```python
from build123d import *

# Parameters (mm, degrees)
SKETCH_1_R       = 1.25
BOARD_DEPTH      = 1
SKETCH_2_W       = 37.3
SKETCH_2_H       = 30
SCREEN_DEPTH     = 2
SCREEN_RADIUS_R  = 3.5
SKETCH_3_W       = 51
SKETCH_3_H       = 5
PLUG_DEPTH       = 7
SKETCH_4_W       = 15.14
SKETCH_4_H       = 20
SPEAKER_DEPTH    = 5
SKETCH_5_W       = 4.5
SKETCH_5_H       = 2.5
BUTTON_DEPTH     = 3.4
SKETCH_6_R       = 1
BUTTON_TAP_DEPTH = 0.5


with BuildPart() as part:
    # 草图1 → board (new body)
    with BuildSketch(Plane(origin=(0, 0, 0), x_dir=(1, 0, 0), z_dir=(0, 1, 0))):
        with BuildLine():
            Line((-29.5, 15), (29.5, 15))
            ThreePointArc((29.5, 15), (31.621320344, 14.121320344), (32.5, 12))
            Line((32.5, 12), (32.5, -12))
            ThreePointArc((32.5, -12), (31.621320344, -14.121320344), (29.5, -15))
            Line((29.5, -15), (-29.5, -15))
            ThreePointArc((-29.5, -15), (-31.621320344, -14.121320344), (-32.5, -12))
            Line((-32.5, -12), (-32.5, 12))
            ThreePointArc((-32.5, 12), (-31.621320344, 14.121320344), (-29.5, 15))
        make_face()
        with Locations(Location((-29.5, 12, 0), (0, 0, 270))):
            Circle(SKETCH_1_R, mode=Mode.SUBTRACT)
        with Locations(Location((29.5, 12, 0), (0, 0, 270))):
            Circle(SKETCH_1_R, mode=Mode.SUBTRACT)
        with Locations(Location((-29.5, -12, 0), (0, 0, 270))):
            Circle(SKETCH_1_R, mode=Mode.SUBTRACT)
        with Locations(Location((29.5, -12, 0), (0, 0, 270))):
            Circle(SKETCH_1_R, mode=Mode.SUBTRACT)
    extrude(amount=BOARD_DEPTH)

    # 草图2 → screen (add)
    with BuildSketch(Plane(origin=(0, 1, 0), x_dir=(1, 0, 0), z_dir=(0, 1, 0))):
        with Locations((-8.15, 0)):
            Rectangle(SKETCH_2_W, SKETCH_2_H)
    extrude(amount=SCREEN_DEPTH)

    # screen-radius
    screen_radius_edges = [part.edges().sort_by_distance(p)[0] for p in [
        (-26.8, 2, -15),
        (-26.8, 2, 15),
        (10.5, 2, 15),
        (10.5, 2, -15),
    ]]
    fillet(screen_radius_edges, radius=SCREEN_RADIUS_R)

    # 草图3 → plug (add)
    with BuildSketch(Plane.XZ):
        with Locations((0, -11.5)):
            Rectangle(SKETCH_3_W, SKETCH_3_H)
    extrude(amount=PLUG_DEPTH)

    # 草图4 → speaker (add)
    with BuildSketch(Plane.XZ):
        with Locations((18.18, 2.216190629)):
            Rectangle(SKETCH_4_W, SKETCH_4_H)
    extrude(amount=SPEAKER_DEPTH)

    # 草图5 → button (add)
    with BuildSketch(Plane.XZ):
        with Locations((-14.75, 13.25)):
            Rectangle(SKETCH_5_W, SKETCH_5_H)
    extrude(amount=BUTTON_DEPTH)

    # 草图6 → button-tap (add)
    with BuildSketch(Plane.XY.offset(14.5)):
        with Locations(Location((-14.75, -1.7, 0), (0, 0, 180))):
            Circle(SKETCH_6_R)
    extrude(amount=BUTTON_TAP_DEPTH)


solid = part.part
```
Geometry check sheet. Reference: the model listing, model coordinates, mm. A direction names the side the tool comes from. Coordinates: 2 decimals unless noted, no trailing zeros. Write each loop counter-clockwise with the first axis right and the second up, starting at its lowest first coordinate (ties: lowest second). Pieces come first, ordered by that corner, then holes. Notation, with made-up numbers: M 66.25,78 L 111.25,78 A29 cw 111.25,101 Z; hole C -36,54.5 d3. An arc over 180 degrees is marked long. One line per item, written item: value. Start each with the question number.
(1) Tool access check on faces 1 (the face through (-26.8, 2, 0)), 2 (the face through (9.45, 2.01, 14)), 3 (the face through (-16, -2, 14.5)). Record the directions out of +Z, -Z, +X, -X, +Y, -Y that give a thin tool (end or side, any length) a straight path to the whole face; none if there is none.
(2) Depth check by flat-ended pin: pin 1 (2.5 mm diameter, centred on y = -2.5, z = 6, fed in from -X); pin 2 (1 mm diameter, centred on x = 25, y = -1.5, fed in from +Z); pin 3 (1.6 mm diameter, centred on y = 2, z = -3.5, fed in from -X); pin 4 (2 mm diameter, centred on x = -29.5, z = 12, fed in from -Y). Enter the tip coordinate at first touch or a pass-through.
(3) Release check for a two-part mould opening along Z. For faces 4 (the face through (9.45, 2.01, -14)), 5 (the face through (-25.5, -3, -12)), 6 (the face through (-6, 1, 15)), 7 (the face through (-28.655, 0.493, 11.079)) record: released by +Z, released by -Z, zero draft, split by the parting line, or undercut.
(4) Sectioned sample at C-C, the plane z = 4. Enter the section's corners in (x, y), and give its area (3 significant figures).
(5) Sectioned sample at D-D, the plane y = -6.25. Enter the section's corners in (x, z).
(6) Sectioned sample at B-B, the plane x = 15. Enter the section's corners in (y, z), and give its area (3 significant figures).
(7) Scan lines: line 1 along X through (y, z) = (0.6, 12); line 2 along Z through (x, y) = (23.5, -1.5); line 3 along Y through (x, z) = (13, -13). Record each from-to range of solid material in increasing order. Write a range as [from, to].
(8) Sectioned sample at A-A, the plane y = -1.7. Enter the section's corners in (x, z), and give its area (3 significant figures).
Filled sheet:
1. face 1: +Z, -Z, -X, +Y
1. face 2: +Z, +X, +Y
1. face 3: +Z
2. pin 1: x = 10.61
2. pin 2: z = 12.22
2. pin 3: x = -26.8
2. pin 4: through
3. face 4: released by -Z
3. face 5: zero draft
3. face 6: released by +Z
3. face 7: undercut
4. outline: M -32.5,0 L 10.61,0 L 10.61,-5 L 25.75,-5 L 25.75,0 L 32.5,0 L 32.5,1 L 10.5,1 L 10.5,3 L -26.8,3 L -26.8,1 L -32.5,1 Z
4. area: 215 mm²
5. outline: M -25.5,-14 L 25.5,-14 L 25.5,-9 L -25.5,-9 Z
6. outline: M -7,-14 L 0,-14 L 0,-15 L 1,-15 L 1,15 L 0,15 L 0,12.22 L -5,12.22 L -5,-7.78 L 0,-7.78 L 0,-9 L -7,-9 Z
6. area: 165 mm²
7. line 1: [-32.5, -30.75], [-28.25, 28.25], [30.75, 32.5]
7. line 2: [-14, -9], [-7.78, 12.22]
7. line 3: [-7, 1]
8. outline: M -25.5,-14 L 25.5,-14 L 25.5,-9 L -25.5,-9 Z; M -17,12 L -12.5,12 L -12.5,14.5 L -13.75,14.5 L -13.75,15 L -15.75,15 L -15.75,14.5 L -17,14.5 Z; M 10.61,-7.78 L 25.75,-7.78 L 25.75,12.22 L 10.61,12.22 Z
8. area: 570 mm²
